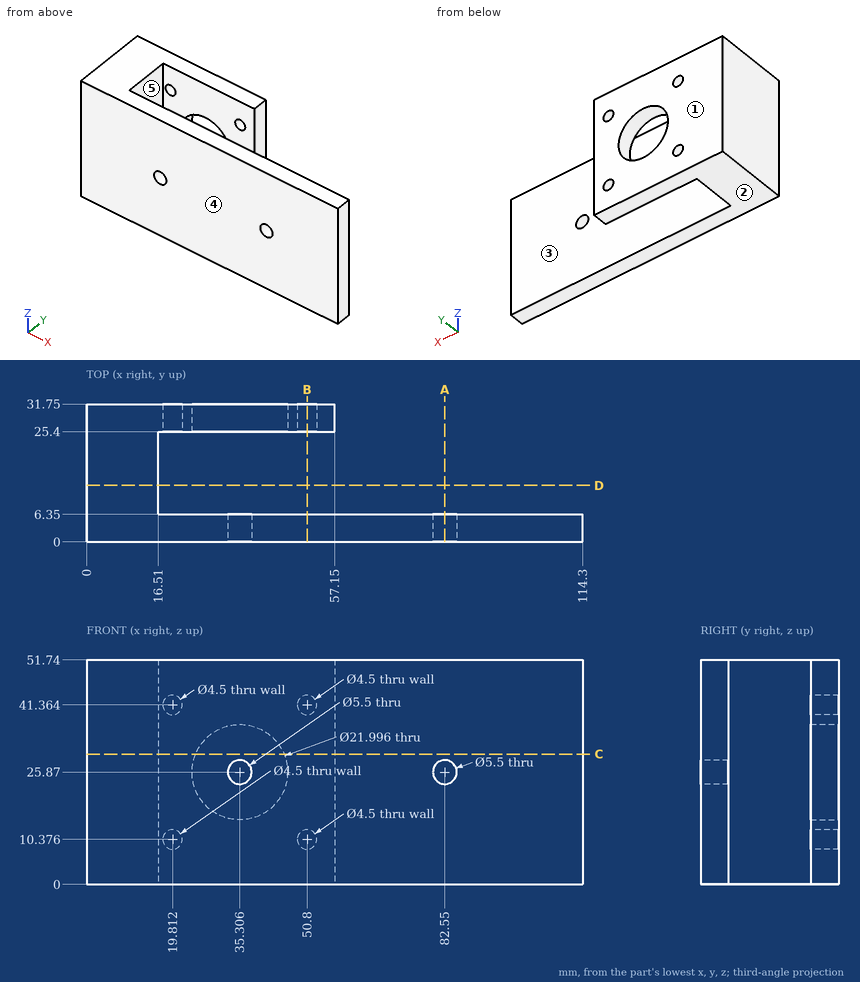
Source: three-view drawing plus pictorial views. Frame: mm from the lowest corner of the part. A direction names the side the tool comes from. Give positions to 0.01 mm unless a question says otherwise; leave off trailing zeros. Order: outer loops, then holes, each group sorted by start corner. A loop starts at its lowest first (then second) coordinate and runs counter-clockwise, first axis right, second up. Notation, with made-up numbers: (-26.5, 5.5) -> (-9.5, 5.5) arc R34 cw to (-9.5, 35.5) -> close; hole circle Ø3 at (56, -19.75). An arc over 180 degrees is marked (long way). Use a Markdown table: item, result.
Q1. First-contact query: P1, Ø5, axis at y = 30, z = 31, coming from the +X side; P2, Ø4, axis at y = 13.5, z = 36, coming from the +X side. Flat tips, straight axial feed; report the tip coordinate or a pass-through.
A:
| item | result |
|---|---|
| P1 | x = 57.15 |
| P2 | x = 16.51 |
Q2. Section B-B (x = 50.8). Return the cut outline in (y, z).
A:
| item | result |
|---|---|
| outline | (0, 0) -> (6.35, 0) -> (6.35, 51.74) -> (0, 51.74) -> close; (25.4, 0) -> (31.75, 0) -> (31.75, 8.13) -> (25.4, 8.13) -> close; (25.4, 12.63) -> (31.75, 12.63) -> (31.75, 39.11) -> (25.4, 39.11) -> close; (25.4, 43.61) -> (31.75, 43.61) -> (31.75, 51.74) -> (25.4, 51.74) -> close |
Q3. Section C-C (z = 30). Return the cut outline in (x, y).
A:
| item | result |
|---|---|
| outline | (0, 0) -> (114.3, 0) -> (114.3, 6.35) -> (16.51, 6.35) -> (16.51, 25.4) -> (25.11, 25.4) -> (25.11, 31.75) -> (0, 31.75) -> close; (45.5, 25.4) -> (57.15, 25.4) -> (57.15, 31.75) -> (45.5, 31.75) -> close |
Q4. Section A-A (x = 82.55). Return the cut outline in (y, z), and give its area (3 significant figures).
A:
| item | result |
|---|---|
| outline | (0, 0) -> (6.35, 0) -> (6.35, 23.12) -> (0, 23.12) -> close; (0, 28.62) -> (6.35, 28.62) -> (6.35, 51.74) -> (0, 51.74) -> close |
| area | 294 mm^2 |
Q5. Section D-D (y = 13). Return the cut outline in (x, z).
A:
| item | result |
|---|---|
| outline | (0, 0) -> (16.51, 0) -> (16.51, 51.74) -> (0, 51.74) -> close |
Q6. Access query for the marked faces 4 and 5. Directions: +Z, -Z, +X, -X, +Y, -Y. A direction counts if a zero-diameter tool reaches every point of the face in a straight line with its end or side. Return the directions, or none.
A:
| item | result |
|---|---|
| face 4 | +Z, -Z, +X, -X, -Y |
| face 5 | +Z, -Z, +X |
Q7. Pull-direction query (Y, two-part tool) for the marked faces 1, 2 and 3; classes: +Y half, -Y half, draft (parallel to the pull), parting line (faces both ways), or undercut.
A:
| item | result |
|---|---|
| face 1 | +Y half |
| face 2 | draft |
| face 3 | undercut |
Q8. Material intervals for line 1 (Z direction, x = 50, y = 29); line 2 (Y direction, x = 45.5, z = 13); line 3 (X direction, y = 4.5, z = 25) (1 decimal), sorted ascending. Write a range as [from, to].
A:
| item | result |
|---|---|
| line 1 | [0, 8.27], [12.48, 39.26], [43.47, 51.74] |
| line 2 | [0, 6.35], [25.4, 31.75] |
| line 3 | [0, 32.7], [37.9, 79.9], [85.2, 114.3] |
